Check sheet for the modelled part. Datum: model origin and axes. Units: mm. A direction names the side the tool comes from. Give positions to 0.01 mm unless a question says otherwise; leave off trailing zeros. Write each loop counter-clockwise with the first axis right and the second up, starting at its lowest first coordinate (ties: lowest second). Pieces come first, ordered by that corner, then holes. Notation, with made-up numbers: M 18.25,-30.5 L 29.25,-30.5 A7 ccw 29.25,-26.5 Z; hole C 32,58 d6. An arc over 180 degrees is marked long. Write item = value, one per line. Start each with the question number.
1) Cross-section at A-A, the plane x = 6. Record the cut outline in (y, z), plus the area to 4 significant figures.
2) Cross-section at C-C, the plane y = 7. Record the cut outline in (x, z).
3) Access from +Z, -Z, +X, -X, +Y, -Y to the whole of each face (thin tool, end or side, straight path). Record for faces 1 (the flat face through (1, 10, 118)), 2 (the flat face through (0, 10, 118)).
4) Cross-section at B-B, the plane z = 151. Record the cut outline in (x, y).
5) Scan lines: line 1 along Z through (x, y) = (6, 0.75); line 2 along X through (y, z) = (0.65, 5); line 3 along X through (y, z) = (12, 227.5). Record each from-to range of solid material in increasing order. Write a range as [from, to].
6) Go/stop test with flat-tipped pins: pin 1 (4 mm diameter, centred on x = 6, z = 235, fed in from -Y); pin 2 (5.5 mm diameter, centred on y = 10, z = 130, fed in from +X); pin 3 (4.5 mm diameter, centred on x = 6, z = 5, fed in from +Y). Record where each tip stops, or that it passes through.
Autodesk Inventor part; units mm, degrees
ref_plane "YZ Plane" through (0, 0, 0) normal (1, 0, 0) x (0, 1, 0)
ref_plane "XZ Plane" through (0, 0, 0) normal (0, 1, 0) x (-1, 0, 0)
ref_plane "XY Plane" through (0, 0, 0) normal (0, 0, 1) x (1, 0, 0)
sketch "スケッチ2" plane through (0, 0, 0) normal (0, 0, 1) x (1, 0, 0)
  line L0 (0, 0) -> (10, 0)
  line L1 (10, 0) -> (10, 1)
  line L2 (10, 1) -> (0, 1)
  line L3 (0, 1) -> (0, 0)
  line L4 (0, 0) -> (1, 0)
  line L5 (1, 0) -> (1, 20)
  line L6 (1, 20) -> (0, 20)
  line L7 (0, 20) -> (0, 0)
  point P0 (1, 1)
  dimension "d0" = 10
  dimension "d1" = 1
  dimension "d2" = 1
  dimension "d3" = 20
extrude "押し出し1" add sketch "スケッチ2" along normal blind 240
sketch "スケッチ3" plane through (1, 1, 0) normal (0, 1, 0) x (1, 0, 0)
  line L0 (9, 0) -> (0, 0)
  line L1 (0, 0) -> (0, -240)
  line L2 (9, 0) -> (9, -240)
  line L3 (9, 0) -> (9, -240)
  line L4 (9, -240) -> (0, -240)
  point P0 (-1, 0)
  point P1 (5, -235)
  point P2 (5, -120)
  point P3 (5, -5)
  point P4 (9, -120)
  dimension "d13" = 5
  dimension "d15" = 4
  dimension "d16" = 0
  dimension "d17" = 4
  dimension "d18" = 5
  dimension "d19" = 4
hole "穴1" at (6, 1, 235) at (6, 1, 120) at (6, 1, 5) direction (0, -1, 0) diameter 3.5 end through all
properties part number "slide_panel_back_stopper"
Reply:
q1.outline = M 0,0 L 1,0 L 1,3.25 L 0,3.25 Z; M 0,6.75 L 1,6.75 L 1,118.25 L 0,118.25 Z; M 0,121.75 L 1,121.75 L 1,233.25 L 0,233.25 Z; M 0,236.75 L 1,236.75 L 1,240 L 0,240 Z
q1.area = 229.5 mm2
q2.outline = M 0,0 L 1,0 L 1,240 L 0,240 Z
q3.face_1 = +Z, -Z, +X, +Y
q3.face_2 = +Z, -Z, -X, +Y, -Y
q4.outline = M 0,0 L 10,0 L 10,1 L 1,1 L 1,20 L 0,20 Z
q5.line_1 = [0, 3.25], [6.75, 118.25], [121.75, 233.25], [236.75, 240]
q5.line_2 = [0, 4.25], [7.75, 10]
q5.line_3 = [0, 1]
q6.pin_1 = 0
q6.pin_2 = 1
q6.pin_3 = 1
